Read the model definition and answer for the solid it produces. Units are mm, in the model's axes. Face numbers are marked on the shaded views. A direction names the side the tool comes from. Coordinates: 2 decimals unless noted, no trailing zeros. Order: outer loops, then holes, each group sorted by start corner. A loop starts at its lowest first (then second) coordinate and runs counter-clockwise, first axis right, second up.
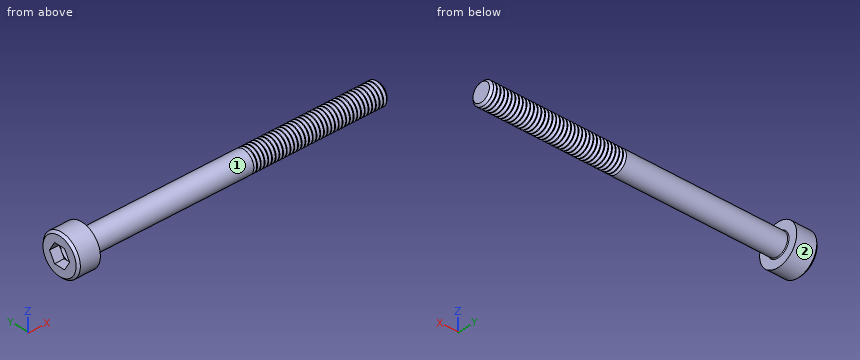
```python
from build123d import *

# Parameters (mm, degrees)
FILLET1_R       = 0.1
HEX_2_DEPTH     = 1.3
THDSCHPAT_COUNT = 37
THDSCHPAT_PITCH = 0.5


with BuildPart() as part:
    # BodySke → Base-Revolve (revolve)
    with BuildSketch(Plane.XY):
        Polygon((0, 0), (0, 2.45), (0.3, 2.75), (3, 2.75), (3, 1.5), (42.7195, 1.5), (43, 1.2195), (43, 0), align=None)
    revolve(axis=Axis((-31.75, 0, 0), (1, 0, 0)))

    # Fillet1
    fillet1_edges = [part.edges().sort_by_distance(p)[0] for p in [
        (3, -1.5, 0),
    ]]
    fillet(fillet1_edges, radius=FILLET1_R)

    # Sketch2 → Hex-PreBroach (revolve, cut)
    with BuildSketch(Plane.XY):
        Polygon((0, 1.28), (1.3, 1.28), (2.039008345, 0), (0, 0), align=None)
    revolve(axis=Axis((0, 0, 0), (1, 0, 0)), mode=Mode.SUBTRACT)

    # Sketch3 → Hex 2 (cut)
    with BuildSketch(Plane(origin=(0, 0, 0), x_dir=(0, 0.5, 0.866025404), z_dir=(-1, 0, 0))):
        Polygon((0.739008345, 1.28), (-0.739008345, 1.28), (-1.478016689, 0), (-0.739008345, -1.28), (0.739008345, -1.28), (1.478016689, 0), align=None)
    extrude(amount=-HEX_2_DEPTH, mode=Mode.SUBTRACT)

    # ThdSchSke → ThreadSchematic (revolve, cut)
    with BuildSketch(Plane.XY):
        Polygon((25, -1.2195), (24.803591786, -1.5), (24.803591786, -1.875), (25.196408214, -1.875), (25.196408214, -1.5), align=None)
    threadschematic = revolve(axis=Axis((-3.175, 0, 0), (1, 0, 0)), mode=Mode.SUBTRACT)

    # ThdSchPat: ThreadSchematic ×37
    with Locations(*[(i * THDSCHPAT_PITCH, 0, 0) for i in range(1, THDSCHPAT_COUNT)]):
        add(threadschematic, mode=Mode.SUBTRACT)


solid = part.part
```
1) Flat-ended cylindrical pins translate along their axes: pin 1 Ø1.5 at (x, y) = (27, 0) entering from -Z; pin 2 Ø0.5 at (y, z) = (0.5, -1) entering from -X; pin 3 Ø1.5 at (x, z) = (6, 1) entering from +Y. Find the tip coordinate at first contact, or state that the pin passes through.
A:
pin 1: stops at z = -1.5
pin 2: stops at x = 1.3
pin 3: stops at y = 1.48
2) Which of the six approach directions +Z, -Z, +X, -X, +Y, -Y give full straight-line access (tool end or side, diameter ignored) to the marked faces 1 and 2?
A:
face 1: +X
face 2: +X, -X
3) Straight lines are drawn through the part: line 1 (Z direction, x = 22.5, y = -1); line 2 (X direction, y = 1.9, z = -1.05); line 3 (Y direction, x = 7.5, z = -0.25). For each, find the intervals that lie inside material, in ascending order.
A:
line 1: z = -1.12 to 1.12
line 2: x = 0 to 3
line 3: y = -1.48 to 1.48
4) A cutting plane is placed at A-A, the plane x = 17. Determine the outline of the cut face in (y, z).
A:
outline: circle Ø3 at (0, 0)
